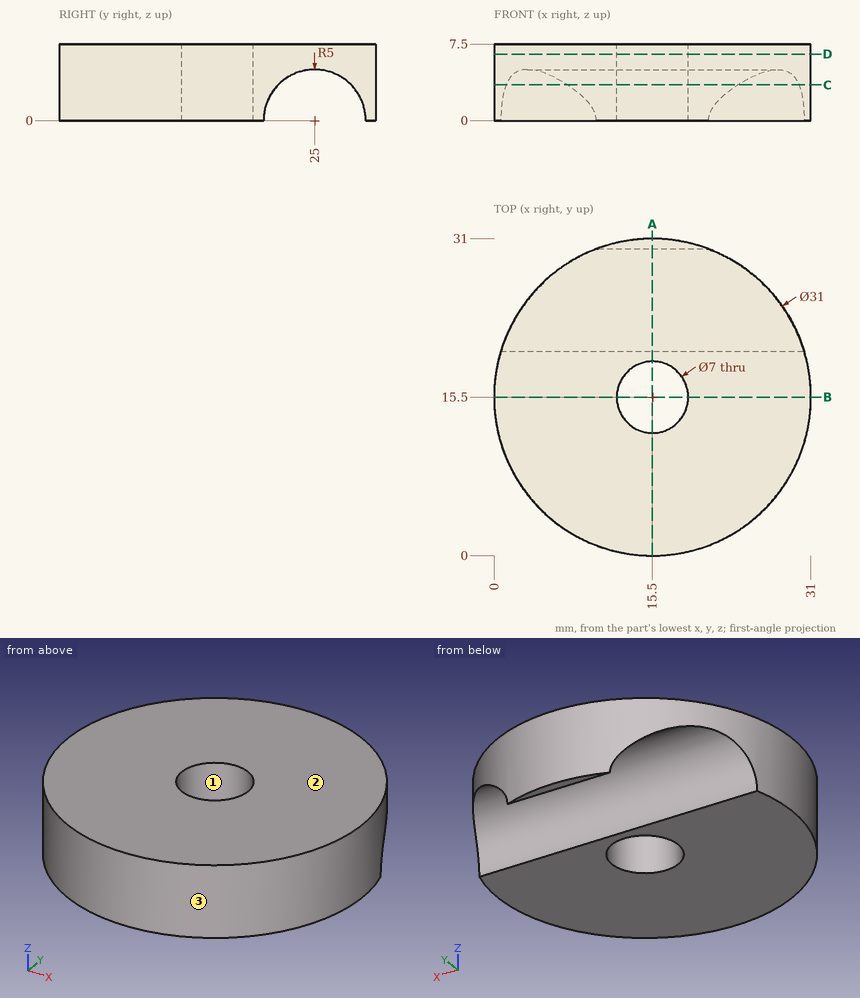
Study the drawing (mm; zero at the part's minimum x, y, z) and answer. Give positions to 0.01 mm unless a question says otherwise; leave off trailing zeros. Write each loop counter-clockwise with the first axis right and the second up, starting at its lowest first coordinate (ties: lowest second). Pieces come first, ordered by that corner, then holes. Notation, with made-up numbers: (-12.75, 59.25) -> (45.25, 59.25) arc R18 ccw to (45.25, 76.25) -> close; hole circle Ø7 at (59.25, 45.5). An arc over 180 degrees is marked (long way). Answer as a JSON object with one key per item and string values. Group by question number.
1) Consider L1, parallel to Y at x = 15.5, z = 2.75; L2, parallel to Y at x = 15.5, z = 5.5; L3, parallel to Y at x = 15.5, z = 1.5. Determine where each line is inside the solid, lowest interval first. Write a range as from..to.
2) Find section B-B (y = 15.5). Write down the section's boundary in (x, z), and give its area (3 significant figures).
3) Each of these flat-tipped pins is pushed along its axis until it touches: P1, Ø5.5, axis at x = 15.5, y = 15.5, coming from the +Z side; P2, Ø4, axis at x = 10, z = 4, coming from the -Y side; P3, Ø1, axis at x = 18, z = 6.5, coming from the +Y side. Where does it stop, or does it pass through?
4) The mould has two halves that part along X. Classify the marked faces 1, 2 and 3: +X half, -X half, draft (parallel to the pull), parting line (faces both ways), or undercut.
5) Find section C-C (z = 3.5). Write down the section's boundary in (x, y), and give its area (3 significant figures).
6) Find section A-A (x = 15.5). Write down the section's boundary in (y, z), and give its area (3 significant figures).
7) Find section D-D (z = 6.5). Write down the section's boundary in (x, y), and give its area (3 significant figures).
Values follow:
{
 "1": {"L1": "y = 0..12, 19..20.82, 29.18..31", "L2": "y = 0..12, 19..31", "L3": "y = 0..12, 19..20.23, 29.77..31"},
 "2": {"outline": "(0, 0) -> (12, 0) -> (12, 7.5) -> (0, 7.5) -> close; (19, 0) -> (31, 0) -> (31, 7.5) -> (19, 7.5) -> close", "area": "180 mm2"},
 "3": {"P1": "passes through", "P2": "stops at y = 0.4", "P3": "stops at y = 30.87"},
 "4": {"face 1": "undercut", "face 2": "draft", "face 3": "parting line"},
 "5": {"outline": "(1.18, 21.43) arc R15.5 ccw (long way) to (29.82, 21.43) -> close; (7.17, 28.57) -> (23.83, 28.57) arc R15.5 ccw to start; hole circle Ø7 at (15.5, 15.5)", "area": "546 mm2"},
 "6": {"outline": "(0, 0) -> (12, 0) -> (12, 7.5) -> (0, 7.5) -> close; (19, 0) -> (20, 0) arc R5 cw to (30, 0) -> (31, 0) -> (31, 7.5) -> (19, 7.5) -> close", "area": "141 mm2"},
 "7": {"outline": "circle Ø31 at (15.5, 15.5); hole circle Ø7 at (15.5, 15.5)", "area": "716 mm2"}
}
